from build123d import *

# Parameters (mm, degrees)
SKETCH2_W         = 34.925
SKETCH2_H         = 3.7846
SLOT_DEPTH        = 8.9662
CIRPATTERN1_COUNT = 2
CIRPATTERN1_ANGLE = 90


with BuildPart() as part:
    # BodySke → Base-Revolve (revolve)
    with BuildSketch(Plane.XY, mode=Mode.PRIVATE) as base_revolve_sk:
        with BuildLine():
            Line((0, 0), (69.050150768, 0))
            Line((69.050150768, 0), (69.050150768, 9.525))
            Line((69.050150768, 9.525), (14.6812, 9.525))
            Line((14.6812, 9.525), (5.550150768, 17.4625))
            ThreePointArc((5.550150768, 17.4625), (1.420913597, 9.161646683), (0, 0))
        make_face()
    revolve(base_revolve_sk.sketch.rotate(Axis((-15.875, 0, 0), (1, 0, 0)), 90), axis=Axis((-15.875, 0, 0), (1, 0, 0)))

    # Sketch2 → Slot (cut)
    with BuildSketch(Plane(origin=(0, 0, 0), x_dir=(0, 0, -1), z_dir=(1, 0, 0))):
        Rectangle(SKETCH2_W, SKETCH2_H)
    extrude(amount=SLOT_DEPTH, mode=Mode.SUBTRACT)

    # Sketch3 → Cross section 0
    with BuildSketch(Plane(origin=(0, 0, 0), x_dir=(0, 0, -1), z_dir=(1, 0, 0))):
        with BuildLine():
            Line((1.3208, -8.3312), (-1.3208, -8.3312))
            Line((-1.3208, -8.3312), (-1.3208, 8.3312))
            Line((-1.3208, 8.3312), (1.3208, 8.3312))
            Line((1.3208, 8.3312), (1.3208, -8.3312))
        make_face()
    # Sketch4 → Cross section 1
    with BuildSketch(Plane(origin=(10.16, 0, 0), x_dir=(0, 0, -1), z_dir=(1, 0, 0))):
        with BuildLine():
            Line((0.6604, -0.6604), (-0.6604, -0.6604))
            Line((-0.6604, -0.6604), (-0.6604, 0.6604))
            Line((-0.6604, 0.6604), (0.6604, 0.6604))
            Line((0.6604, 0.6604), (0.6604, -0.6604))
        make_face()
    cross = loft(mode=Mode.SUBTRACT)

    # CirPattern1: Cross ×2 about axis
    cirpattern1_axis = Axis((0, 0, 0), (1, 0, 0))
    for i in range(1, CIRPATTERN1_COUNT):
        add(cross.rotate(cirpattern1_axis, i * CIRPATTERN1_ANGLE / (CIRPATTERN1_COUNT - 1)), mode=Mode.SUBTRACT)


solid = part.part
Can you work these out from the model? Positions are in its coordinate system, mm. A direction names the side the tool comes from. Give positions to 0.01 mm unless a question says otherwise; leave off trailing zeros. Order: outer loops, then holes, each group sorted by start corner. A loop starts at its lowest first (then second) coordinate and runs counter-clockwise, first axis right, second up. Notation, with made-up numbers: M -18.75,-6.5 L 5.25,-6.5 A25 cw 5.25,32.5 Z; hole C -3.5,79 d5. An arc over 180 degrees is marked long. One line per item, written item: value.
Item 1: If we section it at A-A on x = 30.5: Write out the boundary of the cut face in (y, z) (3 decimals), and give its area (3 significant figures).
Verdict:
outline: C 0,0 d19.05
area: 285 mm2
Item 2: If we mould it in two halves opening along Z, with no side actions, what happens to faces 4 (the face through (10.16, 0, 0)), 5 (the face through (5, 1.892, 4)), 6 (the face through (14.11, -3.01, 9.56))? For each: pulls with the +Z half, pulls with the -Z half, needs draft (parallel to the pull), parting line crosses it, or undercut.
Verdict:
face 4: undercut
face 5: needs draft
face 6: parting line crosses it
Item 3: For faces 1 (the face through (8.966, 0, 3)), 2 (the face through (41.49, 9.3, -2.06)), 3 (the face through (69.05, 0, 0)), which set-ups out of +Z, -Z, +X, -X, +Y, -Y let a thin tool reach every point of the face, with its end or its side?
Verdict:
face 1: +Z, -Z, -X
face 2: +X
face 3: +Z, -Z, +X, +Y, -Y
Item 4: Please list where these lines run through material, in increasing order: line 1 (X direction, y = -2, z = -6); line 2 (Y direction, x = 6, z = -15); line 3 (Y direction, x = 16, z = 8.5).
Verdict:
line 1: 0.67 to 69.05
line 2: -8.15 to -1.89, 1.89 to 8.15
line 3: -4.3 to 4.3
Item 5: For pin 1 (6 mm diameter, centred on y = -1.5, z = -6, fed in from -X); pin 2 (2 mm diameter, centred on x = 49, y = 5.5, fed in from +Z) (3 decimals); pin 3 (5 mm diameter, centred on y = -2.5, z = -6, fed in from -X), each with a flat end and sliding along its axis, tell me the tip position at first contact or that it passes through.
Verdict:
pin 1: x = 0.21
pin 2: z = 8.395
pin 3: x = 0.27
